Could you check a few things on this model? Use its own coordinates, in mm. Face numbers are marked on the shaded views. A direction names the side the tool comes from. Give positions to 0.01 mm unless a question says otherwise; leave off trailing zeros.
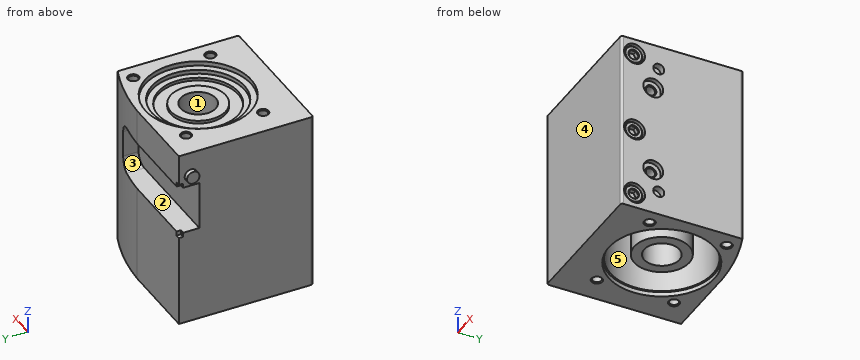
Autodesk Inventor part; units mm, degrees
ref_plane "AXIAL_R_H_XY" through (35, 34, 0) normal (0, 0, 1) x (1, 0, 0)
ref_plane "AXIAL_R_H_YZ" through (35, 34, 0) normal (1, 0, 0) x (0, 1, 0)
ref_plane "AXIAL_R_H_ZX" through (35, 34, 0) normal (0, 1, 0) x (0, 0, 1)
sketch "Sketch_28" plane through (0, 0, 0) normal (0, 0, 1) x (1, 0, 0)
  line L0 (0, 61) -> (0, 0)
  line L1 (0, 0) -> (65, 0)
  line L2 (65, 0) -> (65, 55)
  arc A0 (65, 55) -> (36.5, 61) centre (32.036, -30.8916) ccw
  line L3 (36.5, 61) -> (0, 61)
extrude "Extrusion1" add sketch "Sketch_28" along normal blind 82
sketch "Sketch_20" plane through (0, 0, 0) normal (0, 0, 1) x (1, 0, 0)
  line L0 (-2, 5) -> (-2, -1)
  line L1 (-2, -1) -> (66, -1)
  line L2 (66, -1) -> (66, 57)
  line L3 (66, 57) -> (64, 57)
  line L4 (64, 57) -> (64, 55.4781)
  arc A0 (64.4301, 55.2752) -> (64, 55.4781) centre (38.6219, 1.1094) ccw
  arc A1 (65, 54.3725) -> (64.4301, 55.2752) centre (64, 54.3725) ccw
  line L5 (65, 54.3725) -> (65, 1)
  arc A2 (64, 0) -> (65, 1) centre (64, 1) ccw
  line L6 (64, 0) -> (1, 0)
  arc A3 (0, 1) -> (1, 0) centre (1, 1) ccw
  line L7 (0, 1) -> (0, 5)
  line L8 (0, 5) -> (-2, 5)
extrude "Extrusion2" cut sketch "Sketch_20" along normal blind 82
sketch "Sketch3" plane through (0, 0, 82) normal (0, 0, 1) x (1, 0, 0)
  point P0 (12, 16.5)
hole "Hole1" at (12, 16.5, 82) direction (0, 0, -1) diameter 4.134 depth 13 tip angle 120 countersink diameter 5 countersink angle 90
sketch "Sketch4" plane through (0, 0, 82) normal (0, 0, 1) x (1, 0, 0)
  point P0 (12, 51.5)
hole "Hole2" at (12, 51.5, 82) direction (0, 0, -1) diameter 4.134 depth 13 tip angle 120 countersink diameter 5 countersink angle 90
sketch "Sketch5" plane through (0, 0, 0) normal (0, 0, -1) x (-1, 0, 0)
  point P0 (-12, 16.5)
hole "Hole3" at (12, 16.5, 0) direction (0, 0, 1) diameter 4.134 depth 13 tip angle 120 countersink diameter 5 countersink angle 90
sketch "Sketch6" plane through (0, 0, 0) normal (0, 0, -1) x (-1, 0, 0)
  point P0 (-12, 51.5)
hole "Hole4" at (12, 51.5, 0) direction (0, 0, 1) diameter 4.134 depth 13 tip angle 120 countersink diameter 5 countersink angle 90
sketch "Sketch7" plane through (0, 0, 82) normal (0, 0, 1) x (1, 0, 0)
  point P0 (58, 16.5)
hole "Hole5" at (58, 16.5, 82) direction (0, 0, -1) diameter 4.134 depth 13 tip angle 120 countersink diameter 5 countersink angle 90
sketch "Sketch8" plane through (0, 0, 82) normal (0, 0, 1) x (1, 0, 0)
  point P0 (58, 51.5)
hole "Hole6" at (58, 51.5, 82) direction (0, 0, -1) diameter 4.134 depth 13 tip angle 120 countersink diameter 5 countersink angle 90
sketch "Sketch9" plane through (0, 0, 0) normal (0, 0, -1) x (-1, 0, 0)
  point P0 (-58, 16.5)
hole "Hole7" at (58, 16.5, 0) direction (0, 0, 1) diameter 4.134 depth 13 tip angle 120 countersink diameter 5 countersink angle 90
sketch "Sketch10" plane through (0, 0, 0) normal (0, 0, -1) x (-1, 0, 0)
  point P0 (-58, 51.5)
hole "Hole8" at (58, 51.5, 0) direction (0, 0, 1) diameter 4.134 depth 13 tip angle 120 countersink diameter 5 countersink angle 90
sketch "Sketch_13" plane through (0, 0, 0) normal (1, 0, 0) x (0, 1, 0)
  circle A0 centre (55.5, 71) radius 2.85
extrude "Extrusion3" add sketch "Sketch_13" against normal blind 2
sketch "Sketch12" plane through (65, 1, 0) normal (1, 0, 0) x (0, 0, -1)
  point P0 (-71, 16)
hole "Hole9" at (65, 17, 71) direction (-1, 0, 0) diameter 5 depth 3.1
sketch "Sketch13" plane through (65, 1, 0) normal (1, 0, 0) x (0, 0, -1)
  point P0 (-11, 16)
hole "Hole10" at (65, 17, 11) direction (-1, 0, 0) diameter 5 depth 3.1
sketch "Sketch_18" plane through (0, 14.5, 0) normal (0, 1, 0) x (1, 0, 0)
  line L0 (65, -61) -> (50.7066, -61)
  line L1 (50.7066, -61) -> (51.9, -58.933)
  line L2 (51.9, -58.933) -> (62.467, -58.933)
  line L3 (62.467, -58.933) -> (62.9, -58.5)
  line L4 (62.9, -58.5) -> (62.9, -56.5)
  line L5 (62.9, -56.5) -> (65, -56.5)
  line L6 (65, -56.5) -> (65, -61)
  line L7 (65, -61) -> (50.7066, -61)
revolve "Revolution1" cut sketch "Sketch_18" angle 360 about axis through (65, 14.5, 61) along (1, 0, 0)
thread "Thread1"
sketch "Sketch_19" plane through (0, 14.5, 0) normal (0, 1, 0) x (1, 0, 0)
  line L0 (65, -21) -> (50.7066, -21)
  line L1 (50.7066, -21) -> (51.9, -18.933)
  line L2 (51.9, -18.933) -> (62.467, -18.933)
  line L3 (62.467, -18.933) -> (62.9, -18.5)
  line L4 (62.9, -18.5) -> (62.9, -16.5)
  line L5 (62.9, -16.5) -> (65, -16.5)
  line L6 (65, -16.5) -> (65, -21)
  line L7 (65, -21) -> (50.7066, -21)
revolve "Revolution2" cut sketch "Sketch_19" angle 360 about axis through (65, 14.5, 21) along (1, 0, 0)
thread "Thread2"
sketch "Sketch_26" plane through (0, 6, 0) normal (0, 1, 0) x (1, 0, 0)
  line L0 (65, -7) -> (61.9, -7)
  line L1 (61.9, -7) -> (64.3, -4.6)
  line L2 (64.3, -4.6) -> (64.3, -3.25)
  line L3 (64.3, -3.25) -> (63.8, -2.75)
  line L4 (63.8, -2.75) -> (59.3, -2.75)
  line L5 (59.3, -2.75) -> (59.3, -2.25)
  line L6 (59.3, -2.25) -> (65, -2.25)
  line L7 (65, -2.25) -> (65, -7)
  line L8 (65, -7) -> (61.9, -7)
revolve "Revolution3" cut sketch "Sketch_26" angle 360 about axis through (65, 6, 7) along (1, 0, 0)
sketch "Pattern_1_SKETCH_1" plane through (0, 6, 0) normal (0, 1, 0) x (1, 0, 0)
  line L0 (65, -38) -> (61.9, -38)
  line L1 (61.9, -38) -> (64.3, -35.6)
  line L2 (64.3, -35.6) -> (64.3, -34.25)
  line L3 (64.3, -34.25) -> (63.8, -33.75)
  line L4 (63.8, -33.75) -> (59.3, -33.75)
  line L5 (59.3, -33.75) -> (59.3, -33.25)
  line L6 (59.3, -33.25) -> (65, -33.25)
  line L7 (65, -33.25) -> (65, -38)
  line L8 (65, -38) -> (61.9, -38)
sketch "Pattern_1_SKETCH_2" plane through (0, 6, 0) normal (0, 1, 0) x (1, 0, 0)
  line L0 (65, -75) -> (61.9, -75)
  line L1 (61.9, -75) -> (64.3, -72.6)
  line L2 (64.3, -72.6) -> (64.3, -71.25)
  line L3 (64.3, -71.25) -> (63.8, -70.75)
  line L4 (63.8, -70.75) -> (59.3, -70.75)
  line L5 (59.3, -70.75) -> (59.3, -70.25)
  line L6 (59.3, -70.25) -> (65, -70.25)
  line L7 (65, -70.25) -> (65, -75)
  line L8 (65, -75) -> (61.9, -75)
revolve "Revolution4" cut sketch "Pattern_1_SKETCH_1" angle 360 about axis through (65, 6, 38) along (1, 0, 0)
revolve "Revolution5" cut sketch "Pattern_1_SKETCH_2" angle 360 about axis through (65, 6, 75) along (1, 0, 0)
sketch "Sketch_30" plane through (65, 0, 0) normal (1, 0, 0) x (0, 0, -1)
  line L0 (-9, 4.8453) -> (-7, 3.6906)
  line L1 (-7, 3.6906) -> (-5, 4.8453)
  line L2 (-5, 4.8453) -> (-5, 7.1547)
  line L3 (-5, 7.1547) -> (-7, 8.3094)
  line L4 (-7, 8.3094) -> (-9, 7.1547)
  line L5 (-9, 7.1547) -> (-9, 4.8453)
extrude "Extrusion4" cut sketch "Sketch_30" against normal blind 3.2
sketch "Pattern_2_SKETCH_1" plane through (65, 0, 0) normal (1, 0, 0) x (0, 0, -1)
  line L0 (-40, 4.8453) -> (-38, 3.6906)
  line L1 (-38, 3.6906) -> (-36, 4.8453)
  line L2 (-36, 4.8453) -> (-36, 7.1547)
  line L3 (-36, 7.1547) -> (-38, 8.3094)
  line L4 (-38, 8.3094) -> (-40, 7.1547)
  line L5 (-40, 7.1547) -> (-40, 4.8453)
sketch "Pattern_2_SKETCH_2" plane through (65, 0, 0) normal (1, 0, 0) x (0, 0, -1)
  line L0 (-77, 4.8453) -> (-75, 3.6906)
  line L1 (-75, 3.6906) -> (-73, 4.8453)
  line L2 (-73, 4.8453) -> (-73, 7.1547)
  line L3 (-73, 7.1547) -> (-75, 8.3094)
  line L4 (-75, 8.3094) -> (-77, 7.1547)
  line L5 (-77, 7.1547) -> (-77, 4.8453)
extrude "Extrusion5" cut sketch "Pattern_2_SKETCH_1" against normal blind 3.2
extrude "Extrusion6" cut sketch "Pattern_2_SKETCH_2" against normal blind 3.2
sketch "Sketch_27" plane through (0, 51.7, 0) normal (0, 1, 0) x (1, 0, 0)
  line L0 (0, -44) -> (0, -66)
  line L1 (0, -66) -> (48, -66)
  arc A0 (48, -66) -> (53, -61) centre (48, -61) ccw
  line L2 (53, -61) -> (53, -49)
  arc A1 (53, -49) -> (48, -44) centre (48, -49) ccw
  line L3 (48, -44) -> (0, -44)
extrude "Extrusion7" cut sketch "Sketch_27" along normal blind 9.3
sketch "Sketch_24" plane through (0, 0, 0) normal (1, 0, 0) x (0, 1, 0)
  line L0 (59.05, 68) -> (59.05, 42)
  line L1 (59.05, 42) -> (61, 42)
  line L2 (61, 42) -> (61, 68)
  line L3 (61, 68) -> (59.05, 68)
extrude "Extrusion8" cut sketch "Sketch_24" along normal blind 2
sketch "Sketch_32" plane through (35, 0, 0) normal (1, 0, 0) x (0, 0, -1)
  line L0 (0, 34) -> (-82, 34)
  line L1 (-82, 34) -> (-82, 58)
  line L2 (-82, 58) -> (-79.9, 58)
  line L3 (-79.9, 58) -> (-79.9, 55)
  line L4 (-79.9, 55) -> (-78, 55)
  line L5 (-78, 55) -> (-78, 52.15)
  line L6 (-78, 52.15) -> (-76.65, 52.15)
  line L7 (-76.65, 52.15) -> (-76.65, 46.5)
  line L8 (-76.65, 46.5) -> (-78, 46.5)
  line L9 (-78, 46.5) -> (-78, 42)
  line L10 (-78, 42) -> (-51, 42)
  line L11 (-51, 42) -> (-51, 42.8)
  line L12 (-51, 42.8) -> (-31, 42.8)
  line L13 (-31, 42.8) -> (-31, 42)
  line L14 (-31, 42) -> (-4, 42)
  line L15 (-4, 42) -> (-4, 46.5)
  line L16 (-4, 46.5) -> (-31, 46.5)
  line L17 (-31, 46.5) -> (-31, 57.25)
  line L18 (-31, 57.25) -> (-2.1, 57.25)
  line L19 (-2.1, 57.25) -> (-2.1, 58)
  line L20 (-2.1, 58) -> (0, 58)
  line L21 (0, 58) -> (0, 34)
  line L22 (0, 34) -> (-82, 34)
revolve "Revolution6" cut sketch "Sketch_32" angle 360 about axis through (35, 34, 0) along (0, 0, -1)
ref_plane "AXIAL_R_H_XY" through (35, 34, 0) normal (0, 0, 1) x (1, 0, 0)
ref_plane "AXIAL_R_H_YZ" through (35, 34, 0) normal (1, 0, 0) x (0, 1, 0)
ref_plane "AXIAL_R_H_ZX" through (35, 34, 0) normal (0, 1, 0) x (0, 0, 1)
ref_plane "AXIAL_R_V_XY" through (35, 34, 82) normal (0, 0, -1) x (1, 0, 0)
ref_plane "AXIAL_R_V_YZ" through (35, 34, 82) normal (1, 0, 0) x (0, -1, 0)
ref_plane "AXIAL_R_V_ZX" through (35, 34, 82) normal (0, -1, 0) x (0, 0, -1)
ref_plane "CUP1_XY" through (35, 34, 0) normal (0, 0, -1) x (1, 0, 0)
ref_plane "CUP1_YZ" through (35, 34, 0) normal (1, 0, 0) x (0, -1, 0)
ref_plane "CUP1_ZX" through (35, 34, 0) normal (0, -1, 0) x (0, 0, -1)
ref_plane "CUP2_XY" through (35, 34, 82) normal (0, 0, 1) x (1, 0, 0)
ref_plane "CUP2_YZ" through (35, 34, 82) normal (1, 0, 0) x (0, 1, 0)
ref_plane "CUP2_ZX" through (35, 34, 82) normal (0, 1, 0) x (0, 0, 1)
ref_plane "DR_XY" through (0, -0.5, 41) normal (-1, 0, 0) x (0, 0, 1)
ref_plane "DR_YZ" through (0, -0.5, 41) normal (0, 0, 1) x (0, 1, 0)
ref_plane "DR_ZX" through (0, -0.5, 41) normal (0, 1, 0) x (-1, 0, 0)
ref_plane "TO_AK_XY" through (0, 51.7, 55) normal (1, 0, 0) x (0, 0, -1)
ref_plane "TO_AK_YZ" through (0, 51.7, 55) normal (0, 0, -1) x (0, 1, 0)
ref_plane "TO_AK_ZX" through (0, 51.7, 55) normal (0, 1, 0) x (1, 0, 0)
ref_plane "WELLENZAPFEN_R_H_XY" through (35, 34, 4) normal (0, 0, 1) x (1, 0, 0)
ref_plane "WELLENZAPFEN_R_H_YZ" through (35, 34, 4) normal (1, 0, 0) x (0, 1, 0)
ref_plane "WELLENZAPFEN_R_H_ZX" through (35, 34, 4) normal (0, 1, 0) x (0, 0, 1)
ref_plane "WELLENZAPFEN_R_V_XY" through (35, 34, 78) normal (0, 0, -1) x (1, 0, 0)
ref_plane "WELLENZAPFEN_R_V_YZ" through (35, 34, 78) normal (1, 0, 0) x (0, -1, 0)
ref_plane "WELLENZAPFEN_R_V_ZX" through (35, 34, 78) normal (0, -1, 0) x (0, 0, -1)
properties part number "EGC-80-TB-KF___(0_0_Deckel RE)"
Item 1: For the marked faces 1 and 2, which set-ups out of +Z, -Z, +X, -X, +Y, -Y let a thin tool reach every point of the face, with its end or its side?
Findings:
face 1: +Z, -Z
face 2: -X, +Y
Item 2: For pin 1 (5 mm diameter, centred on x = 14.5, y = 7, fed in from -Z); pin 2 (3.5 mm diameter, centred on x = 58, y = 51.5, fed in from +Z); pin 3 (14.5 mm diameter, centred on x = 35, y = 34, fed in from +Z); pin 4 (5 mm diameter, centred on x = 50.5, y = 29, fed in from -Z), each with a flat end and sliding along its axis, tell me the tip position at first contact or that it passes through.
Findings:
pin 1: stops at z = 0
pin 2: stops at z = 68.82
pin 3: passes through
pin 4: stops at z = 31
Item 3: Please list where these lines run through material, in increasing order: line 1 along Z through (x, y) = (26.5, 32); line 2 along Z through (x, y) = (51.5, 15); line 3 along Z through (x, y) = (3, 57).
Findings:
line 1: z = 4 to 31, 51 to 78
line 2: z = 0 to 19.72, 22.28 to 59.72, 62.28 to 82
line 3: z = 0 to 44, 66 to 82
Item 4: We'd pull the mould along Y, two halves only. Please class the marked faces 3, 4 and 5: +Y half, -Y half, draft (parallel to the pull), parting line (faces both ways), or undercut.
Findings:
face 3: draft
face 4: -Y half
face 5: undercut
